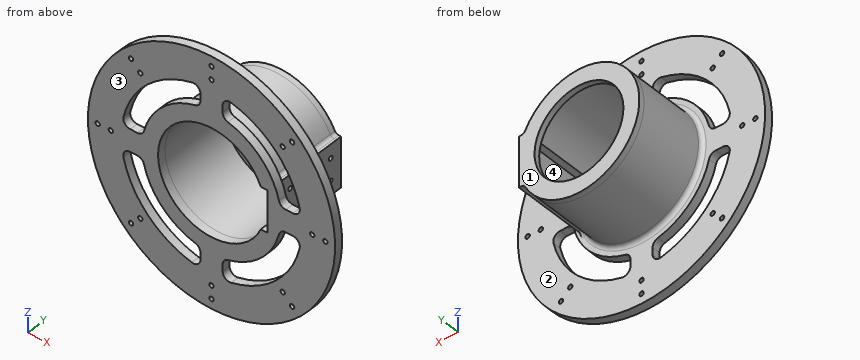
from build123d import *

# Parameters (mm, degrees)
SKETCH1_R           = 75
BOSS_EXTRUDE1_DEPTH = 6
SKETCH3_R           = 32
CUT_EXTRUDE2_DEPTH  = 226.779759943
BOSS_EXTRUDE2_DEPTH = 50
SKETCH5_R           = 1.6
CUT_EXTRUDE3_DEPTH  = 6
SKETCH7_R           = 32
BOSS_EXTRUDE4_DEPTH = 4
CUT_EXTRUDE4_DEPTH  = 6
FILLET1_R           = 3
SKETCH10_R          = 89
SKETCH10_R_2        = 75
SKETCH10_R_3        = 1.6
BOSS_EXTRUDE6_DEPTH = 6
SKETCH11_R          = 1.6
CUT_EXTRUDE6_DEPTH  = 6
FILLET3_R           = 5


with BuildPart() as part:
    # Sketch1 → Boss-Extrude1 (new body)
    with BuildSketch(Plane(origin=(0, 0, 0), x_dir=(1, 0, 0), z_dir=(0, 1, 0))):
        with Locations(Location((105.5, 60.5, 0), (0, 0, 270))):
            Circle(SKETCH1_R)
    extrude(amount=BOSS_EXTRUDE1_DEPTH)

    # Sketch3 → Cut-Extrude2 (cut, through all)
    with BuildSketch(Plane(origin=(0, 6, 0), x_dir=(1, 0, 0), z_dir=(0, 1, 0))):
        with Locations(Location((105.5, 60.5, 0), (0, 0, 270))):
            Circle(SKETCH3_R)
    extrude(amount=-CUT_EXTRUDE2_DEPTH, mode=Mode.SUBTRACT)

    # Sketch4 → Boss-Extrude2 (add)
    with BuildSketch(Plane(origin=(0, 6, 0), x_dir=(1, 0, 0), z_dir=(0, 1, 0))):
        with BuildLine():
            ThreePointArc((140.957721303, 45.5), (67, 60.5), (140.957721303, 75.5))
            Line((140.957721303, 75.5), (145.775366264, 75.5))
            Line((145.775366264, 75.5), (146.331972766, 75.5))
            ThreePointArc((146.331972766, 75.5), (145.74451839, 77.011472968), (145.101136347, 78.5))
            ThreePointArc((145.101136347, 78.5), (62, 60.5), (145.101136347, 42.5))
            ThreePointArc((145.101136347, 42.5), (145.74451839, 43.988527032), (146.331972766, 45.5))
            Line((146.331972766, 45.5), (145.775366264, 45.5))
            Line((145.775366264, 45.5), (140.957721303, 45.5))
        make_face()
        with BuildLine():
            Line((146.331972766, 75.5), (145.775366264, 75.5))
            Line((145.775366264, 75.5), (145.775366264, 45.5))
            Line((145.775366264, 45.5), (146.331972766, 45.5))
            ThreePointArc((146.331972766, 45.5), (147.885391427, 50.715900981), (148.775366264, 56.084949069))
            Line((148.775366264, 56.084949069), (148.775366264, 64.915050931))
            ThreePointArc((148.775366264, 64.915050931), (147.885391427, 70.284099019), (146.331972766, 75.5))
        make_face()
        with BuildLine():
            ThreePointArc((145.101136347, 78.5), (145.74451839, 77.011472968), (146.331972766, 75.5))
            Line((146.331972766, 75.5), (148.775366264, 75.5))
            Line((148.775366264, 75.5), (148.775366264, 78.5))
            Line((148.775366264, 78.5), (145.101136347, 78.5))
        make_face()
        with BuildLine():
            Line((148.775366264, 75.5), (146.331972766, 75.5))
            ThreePointArc((146.331972766, 75.5), (147.885391427, 70.284099019), (148.775366264, 64.915050931))
            Line((148.775366264, 64.915050931), (148.775366264, 75.5))
        make_face()
        with BuildLine():
            ThreePointArc((148.775366264, 56.084949069), (147.885391427, 50.715900981), (146.331972766, 45.5))
            Line((146.331972766, 45.5), (148.775366264, 45.5))
            Line((148.775366264, 45.5), (148.775366264, 56.084949069))
        make_face()
        with BuildLine():
            Line((148.775366264, 45.5), (146.331972766, 45.5))
            ThreePointArc((146.331972766, 45.5), (145.74451839, 43.988527032), (145.101136347, 42.5))
            Line((145.101136347, 42.5), (148.775366264, 42.5))
            Line((148.775366264, 42.5), (148.775366264, 45.5))
        make_face()
    extrude(amount=BOSS_EXTRUDE2_DEPTH)

    # Sketch5 → Cut-Extrude3 (cut)
    with BuildSketch(Plane(origin=(148.775366264, 0, 0), x_dir=(0, 0, -1), z_dir=(1, 0, 0))):
        with Locations((52.5, 51)):
            Circle(SKETCH5_R)
        with Locations((68.5, 51)):
            Circle(SKETCH5_R)
        with Locations((68.5, 16)):
            Circle(SKETCH5_R)
        with Locations((52.5, 16)):
            Circle(SKETCH5_R)
    extrude(amount=-CUT_EXTRUDE3_DEPTH, mode=Mode.SUBTRACT)

    # Sketch7 → Boss-Extrude4 (add)
    with BuildSketch(Plane(origin=(0, 56, 0), x_dir=(1, 0, 0), z_dir=(0, 1, 0))):
        with BuildLine():
            Line((145.101136347, 78.5), (148.775366264, 78.5))
            Line((148.775366264, 78.5), (148.775366264, 42.5))
            Line((148.775366264, 42.5), (145.101136347, 42.5))
            ThreePointArc((145.101136347, 42.5), (62, 60.5), (145.101136347, 78.5))
        make_face()
        with Locations(Location((105.5, 60.5, 0), (0, 0, 270))):
            Circle(SKETCH7_R, mode=Mode.SUBTRACT)
    extrude(amount=BOSS_EXTRUDE4_DEPTH)

    # Sketch8 → Cut-Extrude4 (cut)
    with BuildSketch(Plane.XZ):
        with BuildLine():
            Line((140.957721303, -45.5), (145.775366264, -45.5))
            Line((145.775366264, -45.5), (145.775366264, -75.5))
            Line((145.775366264, -75.5), (140.957721303, -75.5))
            ThreePointArc((140.957721303, -75.5), (67, -60.5), (140.957721303, -45.5))
        make_face()
    extrude(amount=-CUT_EXTRUDE4_DEPTH, mode=Mode.SUBTRACT)

    # Fillet1
    fillet1_edges = [part.edges().sort_by_distance(p)[0] for p in [
        (146.938251306, 6, -42.5),
        (145.101136347, 31, -42.5),
        (62, 6, -60.5),
        (145.101136347, 31, -78.5),
        (146.938251306, 6, -78.5),
    ]]
    fillet(fillet1_edges, radius=FILLET1_R)

    # Sketch10 → Boss-Extrude6 (add)
    with BuildSketch(Plane.XZ):
        with Locations(Location((105.5, -60.5, 0), (0, 0, 270))):
            Circle(SKETCH10_R)
        with Locations((105.5, -60.5)):
            Circle(SKETCH10_R_2, mode=Mode.SUBTRACT)
        with Locations(Location((105.5, 21.5, 0), (0, 0, 270))):
            Circle(SKETCH10_R_3, mode=Mode.SUBTRACT)
        with Locations(Location((163.482756057, -2.517243943, 0), (0, 0, 270))):
            Circle(SKETCH10_R_3, mode=Mode.SUBTRACT)
        with Locations(Location((187.5, -60.5, 0), (0, 0, 270))):
            Circle(SKETCH10_R_3, mode=Mode.SUBTRACT)
        with Locations(Location((163.482756057, -118.482756057, 0), (0, 0, 270))):
            Circle(SKETCH10_R_3, mode=Mode.SUBTRACT)
        with Locations(Location((105.5, -142.5, 0), (0, 0, 270))):
            Circle(SKETCH10_R_3, mode=Mode.SUBTRACT)
        with Locations(Location((47.517243943, -118.482756057, 0), (0, 0, 270))):
            Circle(SKETCH10_R_3, mode=Mode.SUBTRACT)
        with Locations(Location((23.5, -60.5, 0), (0, 0, 270))):
            Circle(SKETCH10_R_3, mode=Mode.SUBTRACT)
        with Locations(Location((47.517243943, -2.517243943, 0), (0, 0, 270))):
            Circle(SKETCH10_R_3, mode=Mode.SUBTRACT)
    extrude(amount=-BOSS_EXTRUDE6_DEPTH)

    # Sketch11 → Cut-Extrude6 (cut)
    with BuildSketch(Plane.XZ):
        with BuildLine():
            ThreePointArc((97.5, -11.144149283), (70.144660941, -25.144660941), (56.144149283, -52.5))
            Line((56.144149283, -52.5), (40.994186309, -52.5))
            ThreePointArc((40.994186309, -52.5), (59.538059223, -14.538059223), (97.5, 4.005813691))
            Line((97.5, 4.005813691), (97.5, -11.144149283))
        make_face()
        with BuildLine():
            ThreePointArc((154.855850717, -52.5), (140.855339059, -25.144660941), (113.5, -11.144149283))
            Line((113.5, -11.144149283), (113.5, 4.005813691))
            ThreePointArc((113.5, 4.005813691), (151.461940777, -14.538059223), (170.005813691, -52.5))
            Line((170.005813691, -52.5), (154.855850717, -52.5))
        make_face()
        with BuildLine():
            Line((113.5, -125.005813691), (113.5, -109.855850717))
            ThreePointArc((113.5, -109.855850717), (140.855339059, -95.855339059), (154.855850717, -68.5))
            Line((154.855850717, -68.5), (170.005813691, -68.5))
            ThreePointArc((170.005813691, -68.5), (151.461940777, -106.461940777), (113.5, -125.005813691))
        make_face()
        with BuildLine():
            Line((40.994186309, -68.5), (56.144149283, -68.5))
            ThreePointArc((56.144149283, -68.5), (70.144660941, -95.855339059), (97.5, -109.855850717))
            Line((97.5, -109.855850717), (97.5, -125.005813691))
            ThreePointArc((97.5, -125.005813691), (59.538059223, -106.461940777), (40.994186309, -68.5))
        make_face()
        with Locations(Location((156.765241636, -111.765241636, 0), (0, 0, 270))):
            Circle(SKETCH11_R)
        with Locations(Location((178, -60.5, 0), (0, 0, 270))):
            Circle(SKETCH11_R)
        with Locations(Location((156.765241636, -9.234758364, 0), (0, 0, 270))):
            Circle(SKETCH11_R)
        with Locations(Location((105.5, 12, 0), (0, 0, 270))):
            Circle(SKETCH11_R)
        with Locations(Location((54.234758364, -9.234758364, 0), (0, 0, 270))):
            Circle(SKETCH11_R)
        with Locations(Location((33, -60.5, 0), (0, 0, 270))):
            Circle(SKETCH11_R)
        with Locations(Location((54.234758364, -111.765241636, 0), (0, 0, 270))):
            Circle(SKETCH11_R)
        with Locations(Location((105.5, -133, 0), (0, 0, 270))):
            Circle(SKETCH11_R)
    extrude(amount=-CUT_EXTRUDE6_DEPTH, mode=Mode.SUBTRACT)

    # Fillet3
    fillet3_edges = [part.edges().sort_by_distance(p)[0] for p in [
        (170.005813691, 3, -52.5),
        (113.5, 3, 4.005813691),
        (113.5, 3, -11.144149283),
        (154.855850717, 3, -52.5),
        (170.005813691, 3, -68.5),
        (154.855850717, 3, -68.5),
        (113.5, 3, -109.855850717),
        (113.5, 3, -125.005813691),
        (97.5, 3, -125.005813691),
        (97.5, 3, -109.855850717),
        (56.144149283, 3, -68.5),
        (40.994186309, 3, -68.5),
        (97.5, 3, 4.005813691),
        (40.994186309, 3, -52.5),
        (56.144149283, 3, -52.5),
        (97.5, 3, -11.144149283),
    ]]
    fillet(fillet3_edges, radius=FILLET3_R)


solid = part.part
Could you check a few things on this model? Use its own coordinates, in mm. Face numbers are marked on the shaded views. A direction names the side the tool comes from. Coordinates: 2 decimals unless noted, no trailing zeros. Order: outer loops, then holes, each group sorted by start corner. A loop starts at its lowest first (then second) coordinate and runs counter-clockwise, first axis right, second up. Notation, with made-up numbers: (62, 4.25) - (106, 4.25) arc R38 ccw to (106, 42.25) - close; hole circle Ø2 at (-36, 4.25). An arc over 180 degrees is marked (long way). Answer in a Markdown table with one row per item. Add a question column.
(1) On a 3-axis mill with a long thin cutter (end or side, diameter ignored), from which of +Z, -Z, +X, -X, +Y, -Y can I reach the whole of each face in a straight line? I mean the marked faces 1 and 2. Say none if no direction works.
(2) I need wall thicknesses on L1, parallel to X at y = 3.8, z = -60.5; L2, parallel to Y at x = 148.1, z = -52.5; L3, parallel to Z at x = 105, y = 4. Which ranges of each line are inside material? Lowest first, please.
(3) If we mould it in two halves opening along X, with no side actions, what happens to the marked faces 3 and 4? For each: released by +X, released by -X, zero draft, split by the parting line, or undercut.
(4) Will these pins go through, and if not, where does the flat tip stop? pin 1 (4 mm diameter, centred on x = 54.23, z = -9.23, fed in from +Y); pin 2 (0.9 mm diameter, centred on x = 147.5, y = 57.5, fed in from +Z); pin 3 (1 mm diameter, centred on x = 142.5, y = 38.5, fed in from -Z).
(5) If we section it at B-B, the plane z = -24.5: State how many separate pieces and enclosed holes the cut face has, then the cut area to 3 significant figures.
(6) If we section it at A-A, the plane y = 44: Please give me the cut outline in (x, z).
Results are:
| question | item | result |
|---|---|---|
| 1 | face 1 | +Z, -Z, +X, -X, +Y |
| 1 | face 2 | +Y |
| 2 | L1 | x = 16.5 to 21.9, 25.1 to 31.4, 34.6 to 67, 145.78 to 176.4, 179.6 to 185.9, 189.1 to 194.5 |
| 2 | L2 | y = 0 to 14.4, 17.6 to 49.4, 52.6 to 60 |
| 2 | L3 | z = -149.5 to -144.02, -140.98 to -134.52, -131.48 to -99, -22 to 10.48, 13.52 to 19.98, 23.02 to 28.5 |
| 3 | face 3 | zero draft |
| 3 | face 4 | undercut |
| 4 | pin 1 | stops at y = 6 |
| 4 | pin 2 | stops at z = -42.5 |
| 4 | pin 3 | stops at z = -84.16 |
| 5 | separate pieces | 3 |
| 5 | enclosed holes | 0 |
| 5 | area | 1,860 mm2 |
| 6 | outline | (144.31, -80.15) arc R3 cw to (146.99, -78.5) - (148.78, -78.5) - (148.78, -42.5) - (146.99, -42.5) arc R3 cw to (144.31, -40.85) arc R43.5 ccw (long way) to start; hole (140.96, -75.5) - (145.78, -75.5) - (145.78, -45.5) - (140.96, -45.5) arc R38.5 ccw (long way) to start |
